Source: CAD feature listing. Evaluate the final solid. Frame: model axes, mm. A direction names the side the tool comes from. Round coordinates to 2 decimals unless told otherwise and drop trailing zeros. Loops run counter-clockwise (first coordinate to the right, second up) from the corner with the lowest first, then second, coordinate; pieces in that order, holes last. Notation, with made-up numbers: (28, 60) - (35, 60) arc R26 ccw to (35, 96) - close; hole circle Ø6 at (34.5, 38). An arc over 180 degrees is marked (long way). One line per question, with ' | ' between items.
from build123d import *

# Parameters (mm, degrees)
BOSS_EXTRUDE1_DEPTH          = 13
CUT_EXTRUDE1_DEPTH           = 10
SKETCH3_W                    = 18.25
SKETCH3_H                    = 12.5
CUT_EXTRUDE2_DEPTH           = 1.5
SKETCH7_R                    = 2.25
BOSS_EXTRUDE2_DEPTH          = 1.65
F_3_0_3_DIAMETER_HOLE1_D     = 3
F_3_0_3_DIAMETER_HOLE1_DEPTH = 12.5


with BuildPart() as part:
    # Sketch1 → Boss-Extrude1 (new, symmetric)
    with BuildSketch(Plane(origin=(0, 0, 0), x_dir=(1, 0, 0), z_dir=(0, 1, 0))):
        with BuildLine():
            Line((9, -6.25), (22.25, 1.399891067))
            Line((22.25, 1.399891067), (22.25, 6.25))
            Line((22.25, 6.25), (0, 6.25))
            ThreePointArc((0, 6.25), (-6.25, 0), (0, -6.25))
            Line((0, -6.25), (9, -6.25))
        make_face()
    extrude(amount=BOSS_EXTRUDE1_DEPTH, both=True)

    # Sketch2 → Cut-Extrude1 (cut, symmetric)
    with BuildSketch(Plane(origin=(0, 0, 0), x_dir=(1, 0, 0), z_dir=(0, 1, 0))):
        Polygon((6.25, 4.75), (6.25, 6.25), (-6.25, 6.25), (-6.25, -6.25), (22.25, -6.25), (22.25, 4.75), align=None)
    extrude(amount=CUT_EXTRUDE1_DEPTH, both=True, mode=Mode.SUBTRACT)

    # Sketch3 → Cut-Extrude2 (cut)
    with BuildSketch(Plane(origin=(0, 13, 0), x_dir=(-1, 0, 0), z_dir=(0, 1, 0))):
        with Locations((-2.875, 0)):
            Rectangle(SKETCH3_W, SKETCH3_H)
    cut_extrude2 = extrude(amount=-CUT_EXTRUDE2_DEPTH, mode=Mode.SUBTRACT)

    # Mirror1: Cut-Extrude2 across plane
    add(cut_extrude2.mirror(Plane.ZX), mode=Mode.SUBTRACT)

    # Sketch7 → Boss-Extrude2 (add)
    with BuildSketch(Plane(origin=(0, 11.5, 0), x_dir=(-1, 0, 0), z_dir=(0, 1, 0))):
        with Locations(Location((0, 0, 0), (0, 0, 90))):
            Circle(SKETCH7_R)
    boss_extrude2 = extrude(amount=BOSS_EXTRUDE2_DEPTH)

    # Mirror2: Boss-Extrude2 across plane
    add(boss_extrude2.mirror(Plane.ZX))

    # Ø3.0 (3) Diameter Hole1
    with Locations(Plane(origin=(0, 0, -6.25), x_dir=(-1, 0, 0), z_dir=(0, 0, -1))):
        with Locations((-10.25, 0), (-18.25, 0)):
            Hole(F_3_0_3_DIAMETER_HOLE1_D / 2, depth=F_3_0_3_DIAMETER_HOLE1_DEPTH)


solid = part.part
1. Section query B-B, the plane y = 0. Return loops of the section in (x, z), plus the area to 3 significant figures.
Worked out:
outline: (6.25, -6.25) - (8.75, -6.25) - (8.75, -4.75) - (6.25, -4.75) - close; (11.75, -6.25) - (16.75, -6.25) - (16.75, -4.75) - (11.75, -4.75) - close; (19.75, -6.25) - (22.25, -6.25) - (22.25, -4.75) - (19.75, -4.75) - close | area: 15.0 mm2
2. Contact query for flat-ended pins moving along their axis: P1, Ø3, axis at x = 17.5, z = 1.5, coming from the +Y side; P2, Ø0.8, axis at y = 12.5, z = -3, coming from the -X side; P3, Ø1.6, axis at y = 0.5, z = -5.5, coming from the -X side; P4, Ø3, axis at x = -2, y = -8, coming from the -Z side. Output: stop coordinate, or through.
Worked out:
P1: stops at y = 13 | P2: stops at x = 12 | P3: stops at x = 6.25 | P4: passes through
3. Material intervals for probe 1 along Y at (x, z) = (18.25, -5.5); probe 2 along Y at (x, z) = (10.25, -5.2); probe 3 along Z at (x, y) = (21, 4), sorted ascending.
Worked out:
probe 1: y = -13 to -1.5, 1.5 to 13 | probe 2: y = -11.5 to -1.5, 1.5 to 11.5 | probe 3: z = -6.25 to -4.75
4. Access query for faces 4 (the flat face through (16, 13, -2)), 5 (the flat face through (6.25, 0, -5)), 6 (the flat face through (12, -12, -1)). Directions: +Z, -Z, +X, -X, +Y, -Y. A direction counts if a zero-diameter tool reaches every point of the face in a straight line with its end or side. Return the directions, or none.
Worked out:
face 4: +Z, -Z, +X, +Y | face 5: +Z, -Z, -X | face 6: +Z, -Z, -Y
5. Section query D-D, the plane x = 6.75. Return loops of the section in (y, z).
Worked out:
outline: (-11.5, -6.25) - (11.5, -6.25) - (11.5, 6.25) - (10, 6.25) - (10, -4.75) - (-10, -4.75) - (-10, 6.25) - (-11.5, 6.25) - close
6. Mould query, pull axis X, two halves, no side actions, for faces 1 (the flat face through (3, 11.5, 0)), 2 (the flat face through (4, -11, 6.25)), 3 (the flat face through (22.25, 0, -5)). Classes: released by +X, released by -X, zero draft, split by the parting line, or undercut.
Worked out:
face 1: undercut | face 2: zero draft | face 3: released by +X
7. Section query C-C, the plane z = 2.75. Return loops of the section in (x, y), plus the area to 3 significant figures.
Worked out:
outline: (-5.61, -11.5) - (12, -11.5) - (12, -13) - (15.06, -13) - (15.06, -10) - (-5.61, -10) - close; (-5.61, 10) - (15.06, 10) - (15.06, 13) - (12, 13) - (12, 11.5) - (-5.61, 11.5) - close | area: 71.2 mm2
8. Section query A-A, the plane x = 10.5. Return loops of the section in (y, z), plus the area to 3 significant figures.
Worked out:
outline: (-11.5, -6.25) - (-1.48, -6.25) - (-1.48, -4.75) - (-10, -4.75) - (-10, 5.38) - (-11.5, 5.38) - close; (1.48, -6.25) - (11.5, -6.25) - (11.5, 5.38) - (10, 5.38) - (10, -4.75) - (1.48, -4.75) - close | area: 60.5 mm2
